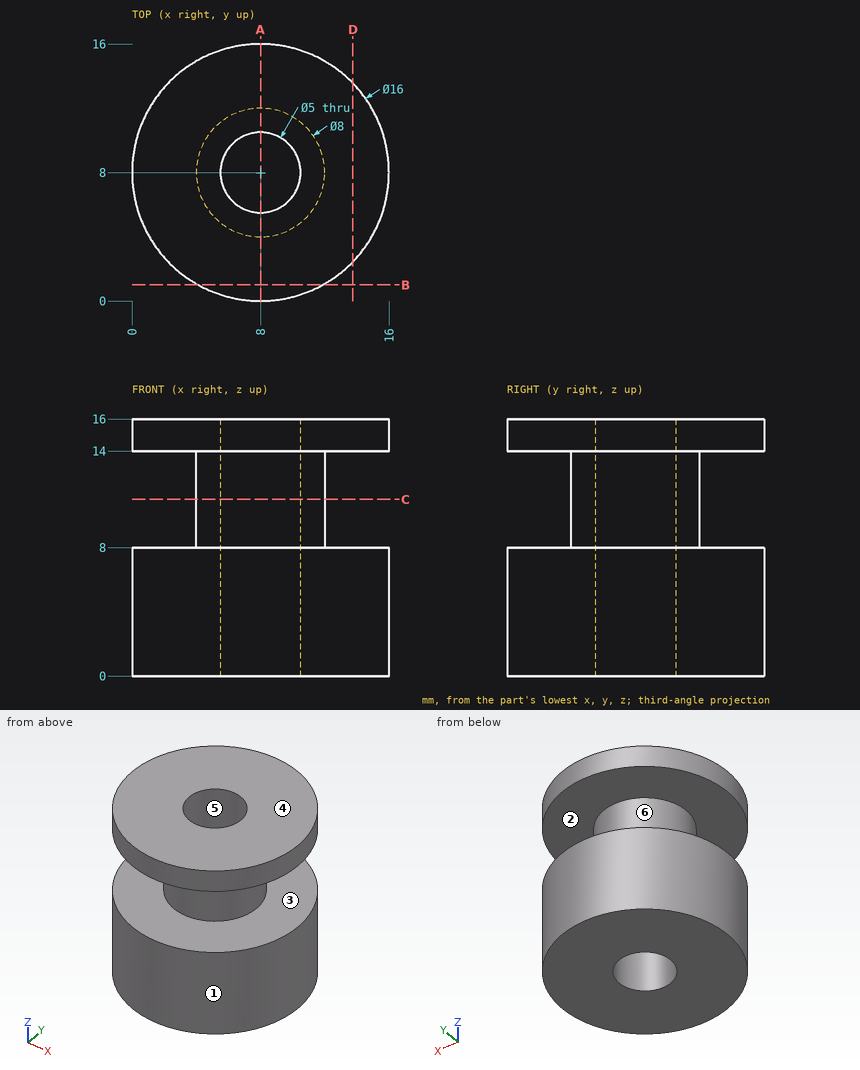
Print and shaded views of the part. All mm, measured from the part's lowest x, y and z. A direction names the side the tool comes from. Coordinates: 2 decimals unless noted, no trailing zeros. Loops run counter-clockwise (first coordinate to the right, second up) from the corner with the lowest first, then second, coordinate; pieces in that order, holes last. Notation, with made-up numbers: (16, 12.5) - (24, 12.5) arc R21 ccw to (24, 47.5) - close; hole circle Ø8 at (-5, 68.5). An arc over 180 degrees is marked (long way). Write item = value, one per line. Start each with the question number.
Item 1: Cut at B-B, the plane y = 1. Give the cut face in (x, z).
Item 2: Cut at A-A, the plane x = 8. Give the cut face in (y, z).
Item 3: Flat gauge pins, fed straight in: pin 1 Ø1 at (y, z) = (5.5, 14) entering from -X; pin 2 Ø1.5 at (x, z) = (4, 12.5) entering from +Y; pin 3 Ø5 at (x, z) = (13.5, 5.5) entering from +Y. Where does each tip first touch, or does it go through?
Item 4: Mould opens along Z. For the marked faces 1, 2, 3 and 4 say: released by +Z, released by -Z, zero draft, split by the parting line, or undercut.
Item 5: 3-axis set-ups, long thin cutter, end or side, ignore diameter. For the marked faces 5 and 6: which of +Z, -Z, +X, -X, +Y, -Y reach the whole face in a straight line?
Item 6: Cut at D-D, the plane x = 13.75. Give the cut face in (y, z).
Item 7: Cut at C-C, the plane z = 11. Give the cut face in (x, y), and give its area (3 significant figures).
Item 8: Wall check: L1, parallel to Z at x = 11.5, y = 12; L2, parallel to Y at x = 8, z = 12.5; L3, parallel to Y at x = 8, z = 3.75. Give the ranges that are in metal, low to high. Write a range as from..to.
The answers:
q1.outline = (4.13, 0) - (11.87, 0) - (11.87, 8) - (4.13, 8) - close; (4.13, 14) - (11.87, 14) - (11.87, 16) - (4.13, 16) - close
q2.outline = (0, 0) - (5.5, 0) - (5.5, 16) - (0, 16) - (0, 14) - (4, 14) - (4, 8) - (0, 8) - close; (10.5, 0) - (16, 0) - (16, 8) - (12, 8) - (12, 14) - (16, 14) - (16, 16) - (10.5, 16) - close
q3.pin_1 = 0.25
q3.pin_2 = 10.33
q3.pin_3 = 15.42
q4.face_1 = zero draft
q4.face_2 = undercut
q4.face_3 = undercut
q4.face_4 = released by +Z
q5.face_5 = +Z, -Z
q5.face_6 = none
q6.outline = (2.44, 0) - (13.56, 0) - (13.56, 8) - (2.44, 8) - close; (2.44, 14) - (13.56, 14) - (13.56, 16) - (2.44, 16) - close
q7.outline = circle Ø8 at (8, 8); hole circle Ø5 at (8, 8)
q7.area = 30.6 mm2
q8.L1 = 0..8, 14..16
q8.L2 = 4..5.5, 10.5..12
q8.L3 = 0..5.5, 10.5..16
